Can you work these out from the model? Positions are in its coordinate system, mm. Give positions to 0.01 mm unless a question says otherwise; leave off trailing zeros. Loops run counter-clockwise (first coordinate to the right, second up) from the corner with the lowest first, then second, coordinate; pieces in that order, holes last. Notation, with made-up numbers: M -4.5,5 L 37.5,5 A20 ccw 37.5,38 Z; hole C -18.75,12.5 d11. An arc over 180 degrees is marked long. Put each result on its own line as item: value. Start each with the question number.
1) Imagine slicing it at B-B (y = 24.5). Write out the boundary of the cut face in (x, z).
2) Please list where these lines run through material, in increasing order: line 1 along X through (y, z) = (73, 9.25); line 2 along Y through (x, z) = (-1.75, -4.25); line 3 along X through (y, z) = (-65.5, -0.5). Write a range as from..to.
3) For P1, Ø3, axis at x = -8, z = -1, coming from the +Y side; P2, Ø4, axis at x = -7, y = 59.5, coming from the +Z side; P3, Ø0.5, axis at x = 0, y = 101.5, coming from the -Z side, each with a flat end and sliding along its axis, tell me the tip position at first contact or that it passes through.
4) Imagine slicing it at A-A (z = 0). Write out the boundary of the cut face in (x, y).
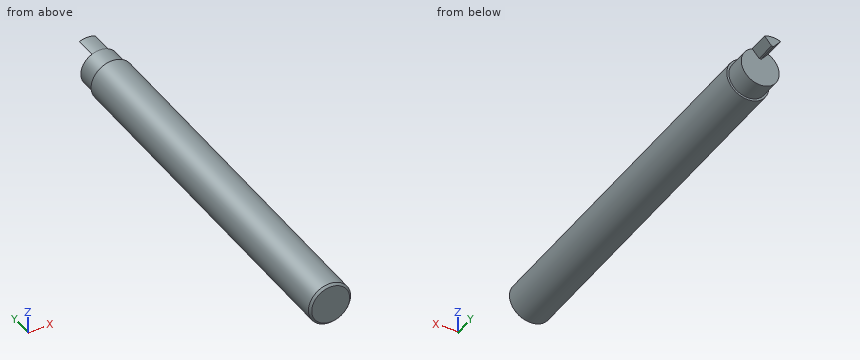
from build123d import *

# Parameters (mm, degrees)
F0_R     = 10
F1_DEPTH = 88.3
F2_R     = 9
F3_DEPTH = 10
F5_DEPTH = 10
F6_SIZE  = 1


with BuildPart() as f1:
    # F0 (on Front) → F1 (new body, symmetric)
    with BuildSketch(Plane.XZ):
        Circle(F0_R)
    extrude(amount=F1_DEPTH, both=True)

    # F2 (on face) → F3 (join)
    with BuildSketch(Plane(origin=(0, 88.3, 0), x_dir=(-1, 0, 0), z_dir=(0, 1, 0))):
        Circle(F2_R)
    extrude(amount=F3_DEPTH)

    # F4 (on face) → F5 (join)
    with BuildSketch(Plane(origin=(0, 98.3, 0), x_dir=(-1, 0, 0), z_dir=(0, 1, 0))):
        with BuildLine():
            ThreePointArc((3.775918, 8.169605), (0, 9), (-3.775918, 8.169605))
            Line((-3.775918, 8.169605), (-0.5, 4.392257))
            Line((-0.5, 4.392257), (0.5, 4.392257))
            Line((0.5, 4.392257), (3.775918, 8.169605))
        make_face()
    extrude(amount=F5_DEPTH)

    # F6
    f6_edges = [f1.edges().sort_by_distance(p)[0] for p in [
        (-10, -88.3, 0),
    ]]
    chamfer(f6_edges, length=F6_SIZE)


solid = f1.part
Recorded:
1. outline: C 0,0 d20
2. line 1: -3.8..3.8
2. line 2: -88.3..98.3
2. line 3: -9.99..9.99
3. P1: y = 98.3
3. P2: z = 8.66
3. P3: z = 4.39
4. outline: M -10,-87.3 L -9,-88.3 L 9,-88.3 L 10,-87.3 L 10,88.3 L 9,88.3 L 9,98.3 L -9,98.3 L -9,88.3 L -10,88.3 Z
